```python
from build123d import *

# Parameters (mm, degrees)
F0_W        = 127
F0_H        = 38.1
F1_DEPTH    = 9.525
F2_R        = 15.875
F3_DEPTH    = 12.7
F5_DEPTH    = 4.7625
F7_DEPTH    = 38.101
F8_T1_DEPTH = 158.75
F8_T3_DEPTH = 95.8787739113
F8_T5_DEPTH = 95.8787739113


# Not quite as in the source:
# - a fillet or chamfer that OpenCascade refuses, or shapes differently, is made with other operations: its cross-section is extruded or revolved along the edge and cut away or added


with BuildPart() as f1:
    # F0 (on Top) → F1 (new body, symmetric)
    with BuildSketch(Plane.XY):
        Rectangle(F0_W, F0_H)
    extrude(amount=F1_DEPTH, both=True)

    # F2 (on face) → F3 (cut)
    with BuildSketch(Plane(origin=(0, 0, -9.525), x_dir=(1, 0, 0), z_dir=(0, 0, -1))):
        with Locations((-44.45, 0)):
            Circle(F2_R)
    extrude(amount=-F3_DEPTH, mode=Mode.SUBTRACT)

    # F4 (on face) → F5 (cut)
    with BuildSketch(Plane(origin=(0, 0, -9.525), x_dir=(1, 0, 0), z_dir=(0, 0, -1))):
        with BuildLine():
            ThreePointArc((-31.2964285714, -8.8881484952), (-17.4248511928, -11.7579152671), (-9.525, 0))
            ThreePointArc((-9.525, 0), (-17.4248511928, 11.7579152671), (-31.2964285714, 8.8881484952))
            ThreePointArc((-31.2964285714, 8.8881484952), (-29.2705966615, 4.6477240974), (-28.575, 0))
            ThreePointArc((-28.575, 0), (-29.2705966615, -4.6477240974), (-31.2964285714, -8.8881484952))
        make_face()
    extrude(amount=-F5_DEPTH, mode=Mode.SUBTRACT)

    # F6 (on face) → F7 (cut, through all)
    with BuildSketch(Plane(origin=(0, 19.05, 0), x_dir=(-1, 0, 0), z_dir=(0, 1, 0))):
        Polygon((31.75, -9.525), (63.5, -9.525), (63.5, -3.175), align=None)
    extrude(amount=-F7_DEPTH, mode=Mode.SUBTRACT)

    # F8: fillet of radius 6.35 on 6 edges, made by hand

    # F8_s2 → F8_t1 (cut)
    with BuildSketch(Plane.YZ.offset(-79.375)):
        with BuildLine():
            ThreePointArc((-12.7, 9.525), (-17.1901280605, 7.6651280605), (-19.05, 3.175))
            Line((-19.05, 3.175), (-19.05, 9.525))
            Line((-19.05, 9.525), (-12.7, 9.525))
        make_face()
        with BuildLine():
            ThreePointArc((19.05, 3.175), (17.1901280605, 7.6651280605), (12.7, 9.525))
            Line((12.7, 9.525), (19.05, 9.525))
            Line((19.05, 9.525), (19.05, 3.175))
        make_face()
        with BuildLine():
            ThreePointArc((-12.7, -9.525), (-17.1901280605, -7.6651280605), (-19.05, -3.175))
            Line((-19.05, -3.175), (-19.05, -9.525))
            Line((-19.05, -9.525), (-12.7, -9.525))
        make_face()
        with BuildLine():
            ThreePointArc((19.05, -3.175), (17.1901280605, -7.6651280605), (12.7, -9.525))
            Line((12.7, -9.525), (19.05, -9.525))
            Line((19.05, -9.525), (19.05, -3.175))
        make_face()
    extrude(amount=F8_T1_DEPTH, mode=Mode.SUBTRACT)

    # F8_s4 → F8_t3 (cut)
    with BuildSketch(Plane(origin=(-76.0138336112, 0, 15.2027667222), x_dir=(0, 1, 0), z_dir=(0.9805806757, 0, -0.1961161351))):
        with BuildLine():
            ThreePointArc((19.05, -9.2167182266), (17.1901280605, -13.7068462871), (12.7, -15.5667182266))
            Line((12.7, -15.5667182266), (19.05, -15.5667182266))
            Line((19.05, -15.5667182266), (19.05, -9.2167182266))
        make_face()
    extrude(amount=F8_T3_DEPTH, mode=Mode.SUBTRACT)

    # F8_s6 → F8_t5 (cut)
    with BuildSketch(Plane(origin=(18.0030392952, 0, -3.600607859), x_dir=(0, 1, 0), z_dir=(-0.9805806757, 0, 0.1961161351))):
        with BuildLine():
            ThreePointArc((-12.7, 15.5667182266), (-17.1901280605, 13.7068462871), (-19.05, 9.2167182266))
            Line((-19.05, 9.2167182266), (-19.05, 15.5667182266))
            Line((-19.05, 15.5667182266), (-12.7, 15.5667182266))
        make_face()
    extrude(amount=F8_T5_DEPTH, mode=Mode.SUBTRACT)


solid = f1.part
```
The listing builds one solid part. Answer for the finished solid, in the listing's coordinates (mm). A direction names the side the tool comes from. Coordinates: 2 decimals unless noted, no trailing zeros. Write each loop counter-clockwise with the first axis right and the second up, starting at its lowest first coordinate (ties: lowest second). Pieces come first, ordered by that corner, then holes. Notation, with made-up numbers: (29.25, 70) - (86.25, 70) arc R20 cw to (86.25, 103) - close; hole circle Ø10 at (-2.75, 67). An arc over 180 degrees is marked (long way). Return JSON: item names as keys, results as strings. Group by question number.
Q1. Find the intervals of material crossed by line 1 along X through (y, z) = (0, -5.5) (3 decimals); line 2 along X through (y, z) = (1, 1); line 3 along X through (y, z) = (6.5, -0.5), in increasing order. Write a range as [from, to].
Q2. Which of the six approach directions +Z, -Z, +X, -X, +Y, -Y give full straight-line access (tool end or side, diameter ignored) to faces 1 (the flat face through (-45, 0, 3.175)), 2 (the cylindrical face through (15.208, -17.14, -7.714))?
Q3. The part is cut by section A-A on x = -0.5. Write down the section's boundary in (y, z) (3 decimals), and give its area (3 significant figures).
Q4. The part is cut by section B-B on y = 0. Write down the section's boundary in (x, z) (1 decimal).
Q5. Flat-ended cylindrical pins translate along their axes: pin 1 Ø6.5 at (x, y) = (-20.5, -5.5) entering from -Z; pin 2 Ø1.5 at (x, y) = (34, 15) entering from -Z; pin 3 Ø9.5 at (x, y) = (-42, -1.5) entering from -Z (3 decimals). Find the tip coordinate at first contact, or state that the pin passes through.
Q6. For a pull along Y with two mould halves and no side action, classify faces 3 (the cylindrical face through (-48.098, 17.239, -4.308)), 4 (the flat face through (13, -19.05, 0)), 5 (the flat face through (-29, -12, -9.525)), 6 (the cylindrical face through (-9.53, 0.42, -7.18)) as +Y half, -Y half, draft (parallel to the pull), parting line (faces both ways), or undercut.
Q7. The part is cut by section C-C on z = 7.75. Write down the section's boundary in (x, y), and give its area (3 significant figures).
Evaluation:
{
 "1": {"line 1": "x = [-9.525, 63.5]", "line 2": "x = [-63.5, -60.29], [-28.61, 63.5]", "line 3": "x = [-63.5, -58.93], [-29.97, 63.5]"},
 "2": {"face 1": "-Z", "face 2": "-Z, +X, -X, -Y"},
 "3": {"outline": "(-19.05, -3.175) arc R6.35 ccw to (-12.7, -9.525) - (12.7, -9.525) arc R6.35 ccw to (19.05, -3.175) - (19.05, 3.175) arc R6.35 ccw to (12.7, 9.525) - (-12.7, 9.525) arc R6.35 ccw to (-19.05, 3.175) - close", "area": "691 mm2"},
 "4": {"outline": "(-63.5, -3.2) - (-60.3, -3.8) - (-60.3, 3.2) - (-28.6, 3.2) - (-28.6, -4.8) - (-9.5, -4.8) - (-9.5, -9.5) - (63.5, -9.5) - (63.5, 9.5) - (-63.5, 9.5) - close"},
 "5": {"pin 1": "stops at z = -4.76", "pin 2": "stops at z = -9.33", "pin 3": "stops at z = 3.175"},
 "6": {"face 3": "+Y half", "face 4": "-Y half", "face 5": "draft", "face 6": "undercut"},
 "7": {"outline": "(-63.5, -17.1) - (63.5, -17.1) - (63.5, 17.1) - (-63.5, 17.1) - close", "area": "4,340 mm2"}
}
